Part model, mm, in its own coordinate system. Face numbers are marked on the shaded views. A direction names the side the tool comes from. Round coordinates to 2 decimals unless told otherwise and drop trailing zeros. Write each loop counter-clockwise with the first axis right and the second up, starting at its lowest first coordinate (ties: lowest second). Pieces come first, ordered by that corner, then holes.
```python
from build123d import *

# Parameters (mm, degrees)
BOSS_EXTRU_1_DEPTH      = 65
ESQUISSE2_W             = 11.96
ESQUISSE2_H             = 28.94
BOSS_EXTRU_2_DEPTH      = 3
ESQUISSE3_W             = 11.96
ESQUISSE3_H             = 8
BOSS_EXTRU_3_DEPTH      = 5
CHANFREIN4_SIZE         = 2
ESQUISSE8_W             = 7.98
ESQUISSE8_H             = 5
ENL_V_MAT_EXTRU_1_DEPTH = 5.96
ESQUISSE9_W             = 3.92
ESQUISSE9_H             = 5
BOSS_EXTRU_5_DEPTH      = 8
BOSS_EXTRU_4_DEPTH      = 8
CONG_2_R                = 0.5
CHANFREIN5_SIZE         = 5


with BuildPart() as part:
    # Esquisse1 → Boss.-Extru.1 (new body)
    with BuildSketch(Plane(origin=(0, 0, 0), x_dir=(1, 0, 0), z_dir=(0, 1, 0))):
        Polygon((7.94, 7.96), (9.97, 7.96), (9.97, 11.94), (1.99, 11.94), (1.99, 7.96), (4.02, 7.96), (4.02, 5.98), (0, 5.98), (0, 0), (11.96, 0), (11.96, 5.98), (7.94, 5.98), align=None)
    extrude(amount=BOSS_EXTRU_1_DEPTH)

    # Esquisse2 → Boss.-Extru.2 (add)
    with BuildSketch(Plane(origin=(0, 65, 0), x_dir=(1, 0, 0), z_dir=(0, 1, 0))):
        with Locations((5.98, 14.47)):
            Rectangle(ESQUISSE2_W, ESQUISSE2_H)
    extrude(amount=BOSS_EXTRU_2_DEPTH)

    # Esquisse3 → Boss.-Extru.3 (add)
    with BuildSketch(Plane(origin=(0, 0, -28.94), x_dir=(-1, 0, 0), z_dir=(0, 0, -1))):
        with Locations((-5.98, 64)):
            Rectangle(ESQUISSE3_W, ESQUISSE3_H)
    extrude(amount=-BOSS_EXTRU_3_DEPTH)

    # Chanfrein4
    chanfrein4_edges = [part.edges().sort_by_distance(p)[0] for p in [
        (1.99, 32.5, -7.96),
        (9.97, 32.5, -7.96),
    ]]
    chamfer(chanfrein4_edges, length=CHANFREIN4_SIZE)

    # Esquisse8 → Enlèv. mat.-Extru.1 (cut)
    with BuildSketch(Plane(origin=(0, 0, -11.94), x_dir=(-1, 0, 0), z_dir=(0, 0, -1))):
        with Locations((-5.98, 62.5)):
            Rectangle(ESQUISSE8_W, ESQUISSE8_H)
    extrude(amount=-ENL_V_MAT_EXTRU_1_DEPTH, mode=Mode.SUBTRACT)

    # Esquisse9 → Boss.-Extru.5 (add)
    with BuildSketch(Plane(origin=(0, 0, -5.98), x_dir=(-1, 0, 0), z_dir=(0, 0, -1))):
        with Locations((-5.98, 62.5)):
            Rectangle(ESQUISSE9_W, ESQUISSE9_H)
    extrude(amount=BOSS_EXTRU_5_DEPTH)

    # Esquisse5 → Boss.-Extru.4 (add)
    with BuildSketch(Plane(origin=(0, 0, -5.98), x_dir=(-1, 0, 0), z_dir=(0, 0, -1))):
        with BuildLine():
            Line((-10.46, 64), (-11.96, 64))
            Line((-11.96, 64), (-11.96, 61))
            Line((-11.96, 61), (-10.46, 61))
            ThreePointArc((-10.46, 61), (-8.96, 62.5), (-10.46, 64))
        make_face()
        with BuildLine():
            Line((-1.5, 61), (0, 61))
            Line((0, 61), (0, 64))
            Line((0, 64), (-1.5, 64))
            ThreePointArc((-1.5, 64), (-3, 62.5), (-1.5, 61))
        make_face()
    extrude(amount=BOSS_EXTRU_4_DEPTH)

    # Congé2
    cong_2_edges = [part.edges().sort_by_distance(p)[0] for p in [
        (2.01, 0, -5.98),
        (2.01, 65, -5.98),
        (4.02, 65, -9.98),
        (7.94, 65, -9.98),
        (4.02, 62.5, -13.98),
        (5.98, 65, -13.98),
        (7.94, 62.5, -13.98),
        (5.98, 60, -13.98),
        (5.98, 0, -11.94),
        (0, 30.5, -5.98),
        (3, 62.5, -5.98),
        (0.75, 61, -5.98),
        (0, 61, -9.98),
        (0.75, 64, -5.98),
        (0, 64, -9.98),
        (3, 62.5, -13.98),
        (0.75, 61, -13.98),
        (0, 62.5, -13.98),
        (0.75, 64, -13.98),
        (11.96, 30.5, -5.98),
        (8.96, 62.5, -5.98),
        (11.21, 64, -5.98),
        (9.95, 0, -5.98),
        (11.96, 64, -9.98),
        (11.21, 61, -5.98),
        (11.96, 61, -9.98),
        (8.96, 62.5, -13.98),
        (11.21, 64, -13.98),
        (11.96, 62.5, -13.98),
        (11.21, 61, -13.98),
        (9.95, 65, -5.98),
        (0, 64.5, -5.98),
        (11.96, 64.5, -5.98),
        (0, 64, -28.94),
        (11.96, 65, -14.96),
        (11.96, 64, -28.94),
        (0, 68, -14.47),
        (11.96, 68, -14.47),
        (5.98, 68, -28.94),
        (0, 65, -14.96),
        (1.99, 30, -11.94),
        (9.97, 30, -11.94),
    ]]
    fillet(cong_2_edges, radius=CONG_2_R - 0.0001)  # a hair under: the kernel refuses the full size

    # Chanfrein5
    chanfrein5_edges = [part.edges().sort_by_distance(p)[0] for p in [
        (5.98, 60, -23.94),
    ]]
    chamfer(chanfrein5_edges, length=CHANFREIN5_SIZE - 0.0001)  # a hair under: the kernel refuses the full size


solid = part.part
```
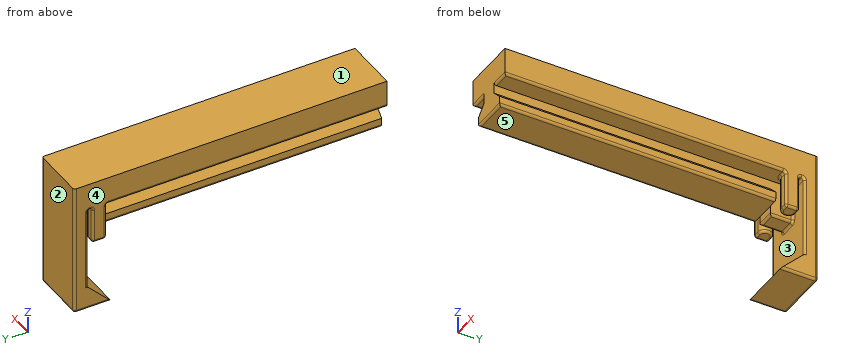
Q1. Drop flat-ended pins along their axis: pin 1 (1 mm diameter, centred on x = 10.5, y = 47, fed in from +Z); pin 2 (1.8 mm diameter, centred on x = 1.5, y = 30, fed in from -Z); pin 3 (1.7 mm diameter, centred on x = 6, z = -12.5, fed in from -Y); pin 4 (4 mm diameter, centred on y = 19, z = -9.5, fed in from +X). Give the stop position or say it passes through.
Values follow:
pin 1: stops at z = 0
pin 2: stops at z = -11.93
pin 3: stops at y = 0.05
pin 4: stops at x = 9.97
Q2. Cut at A-A on z = -10.75. State how many separate pieces and enclosed holes the cut face has, plus the area to 3 significant figures.
Values follow:
separate pieces: 3
enclosed holes: 0
area: 550 mm2
Q3. Cut at D-D on y = 62.5. Write the cut outline in (x, z).
Values follow:
outline: (0, -28.44) arc R0.5 ccw to (0.5, -28.94) - (11.46, -28.94) arc R0.5 ccw to (11.96, -28.44) - (11.96, -26.44) - (0, -26.44) - close; (0, -13.48) arc R0.5 ccw to (0.5, -13.98) - (2.5, -13.98) arc R0.5 ccw to (3, -13.48) - (3, -6.48) arc R0.5 cw to (3.5, -5.98) - (4.02, -5.98) - (4.02, -13.48) arc R0.5 ccw to (4.52, -13.98) - (7.44, -13.98) arc R0.5 ccw to (7.94, -13.48) - (7.94, -5.98) - (8.46, -5.98) arc R0.5 cw to (8.96, -6.48) - (8.96, -13.48) arc R0.5 ccw to (9.46, -13.98) - (11.46, -13.98) arc R0.5 ccw to (11.96, -13.48) - (11.96, 0) - (0, 0) - close
Q4. Wall check: L1, parallel to Z at x = 10, y = 27; L2, parallel to Y at x = 1, z = -20.5; L3, parallel to Z at x = 6.5, y = 49. Give the ranges that are in metal, low to high.
Values follow:
L1: z = -5.98 to 0
L2: y = 65 to 68
L3: z = -11.94 to 0
Q5. Which spindle directions (+Z, -Z, +X, -X, +Y, -Y) get a long thin tool onto all of the face, cutting with end or side? Do the marked faces 4 and 5. Say none if no direction does.
Values follow:
face 4: +Z, -Z, -X, +Y, -Y
face 5: -Z, +X, -X, -Y
Q6. Cut at C-C on z = -21.75. Write the cut outline in (x, y).
Values follow:
outline: (0, 65.5) arc R0.5 ccw to (0.5, 65) - (11.46, 65) arc R0.5 ccw to (11.96, 65.5) - (11.96, 67.5) arc R0.5 ccw to (11.46, 68) - (0.5, 68) arc R0.5 ccw to (0, 67.5) - close
Q7. Mould opens along Y. For the marked faces 1, 2 and 3 say: +Y half, -Y half, draft (parallel to the pull), parting line (faces both ways), or undercut.
Values follow:
face 1: draft
face 2: +Y half
face 3: undercut
